from build123d import *

# Parameters (mm, degrees)
F1_DEPTH       = 260
F3_D           = 11
F3_DEPTH       = 30
F3_CBORE_D     = 19
F3_CBORE_DEPTH = 13
F3_TIP         = 3.3047334047
F4_D           = 8.8
F4_DEPTH       = 30
F4_TIP         = 2.6437867237
F5_D           = 11
F5_DEPTH       = 30
F5_TIP         = 3.3047334047


with BuildPart() as f1:
    # F0 (on Front) → F1 (new body)
    with BuildSketch(Plane.XZ):
        Polygon((100, 23), (0, 23), (0, 0), (95, 0), (95, -5), (100, -5), align=None)
    extrude(amount=-F1_DEPTH)

    # F3
    with Locations(Plane.XY.offset(23)):
        with Locations((14, 239), (86, 239), (14, 187), (86, 187), (86, 73), (86, 21), (14, 73), (14, 21)):
            CounterBoreHole(F3_D / 2, F3_CBORE_D / 2, F3_CBORE_DEPTH, depth=F3_DEPTH)
            with Locations((0, 0, -(F3_DEPTH + F3_TIP / 2))):  # 118° drill point
                Cone(0, F3_D / 2, F3_TIP, mode=Mode.SUBTRACT)

    # F4
    with Locations(Plane.XY.offset(23)):
        with Locations((31, 20), (69, 20), (31, 90), (69, 90), (31, 130), (69, 130)):
            Hole(F4_D / 2, depth=F4_DEPTH)
            with Locations((0, 0, -(F4_DEPTH + F4_TIP / 2))):  # 118° drill point
                Cone(0, F4_D / 2, F4_TIP, mode=Mode.SUBTRACT)

    # F5
    with Locations(Plane.XY.offset(23)):
        with Locations((9, 220), (91, 220), (91, 165), (9, 165)):
            Hole(F5_D / 2, depth=F5_DEPTH)
            with Locations((0, 0, -(F5_DEPTH + F5_TIP / 2))):  # 118° drill point
                Cone(0, F5_D / 2, F5_TIP, mode=Mode.SUBTRACT)


solid = f1.part
Source: CAD feature listing. Evaluate the final solid. Frame: model axes, mm. A direction names the side the tool comes from. Give positions to 0.01 mm unless a question says otherwise; leave off trailing zeros. Order: outer loops, then holes, each group sorted by start corner. A loop starts at its lowest first (then second) coordinate and runs counter-clockwise, first axis right, second up. Notation, with made-up numbers: (-7, 51.5) -> (40, 51.5) arc R24 cw to (40, 84.5) -> close; hole circle Ø7 at (38.5, -33.75). An arc over 180 degrees is marked (long way). Write item = value, one per line.
Item 1: Set-up query: faces 1 (the face through (95.061, 23.854, 16.591)), 2 (the face through (90.4, 183.7, 4.9)). Return all of +Z, -Z, +X, -X, +Y, -Y with unobstructed straight access to the full face (end or side cutting, diameter ignored); none if empty.
Check result:
face_1 = +Z
face_2 = +Z, -Z
Item 2: Mould query, pull axis X, two halves, no side actions, for faces 3 (the face through (100, 128, 9)), 4 (the face through (51, 128, 23)), 5 (the face through (96.495, 220.242, 11.915)). Classes: +X half, -X half, draft (parallel to the pull), parting line (faces both ways), or undercut.
Check result:
face_3 = +X half
face_4 = draft
face_5 = undercut
Item 3: Section query A-A (z = 16.75). State how many separate pieces and enclosed holes the cut face has, then the cut area to 3 significant figures.
Check result:
separate_pieces = 1
enclosed_holes = 18
area = 23,000 mm²
Item 4: Section query C-C (x = 31). Output: boundary loops of the cut face in (y, z), then the cut area to 3 significant figures.
Check result:
outline = (0, 0) -> (15.6, 0) -> (15.6, 23) -> (0, 23) -> close; (24.4, 0) -> (85.6, 0) -> (85.6, 23) -> (24.4, 23) -> close; (94.4, 0) -> (125.6, 0) -> (125.6, 23) -> (94.4, 23) -> close; (134.4, 0) -> (260, 0) -> (260, 23) -> (134.4, 23) -> close
area = 5,370 mm²
Item 5: Ray query, probe 1 along Y at (x, z) = (69, 7.75); probe 2 along X at (y, z) = (88, 9.75); probe 3 along X at (y, z) = (193.5, 21.25). Return the intervals inside material, ascending.
Check result:
probe_1 = 0 to 15.6, 24.4 to 85.6, 94.4 to 125.6, 134.4 to 260
probe_2 = 0 to 27.08, 34.92 to 65.08, 72.92 to 100
probe_3 = 0 to 7.07, 20.93 to 79.07, 92.93 to 100
Item 6: Section query B-B (y = 187). Output: boundary loops of the cut face in (x, z), then the cut area to 3 significant figures.
Check result:
outline = (0, 0) -> (8.5, 0) -> (8.5, 10) -> (4.5, 10) -> (4.5, 23) -> (0, 23) -> close; (19.5, 0) -> (80.5, 0) -> (80.5, 10) -> (76.5, 10) -> (76.5, 23) -> (23.5, 23) -> (23.5, 10) -> (19.5, 10) -> close; (91.5, 0) -> (95, 0) -> (95, -5) -> (100, -5) -> (100, 23) -> (95.5, 23) -> (95.5, 10) -> (91.5, 10) -> close
area = 1,610 mm²
Item 7: Contact query for flat-ended pins moving along their axis: pin 1 (21 mm diameter, centred on x = 10, y = 243, fed in from +Z); pin 2 (8 mm diameter, centred on x = 84, y = 142, fed in from -Z); pin 3 (5.5 mm diameter, centred on x = 89, y = 238.5, fed in from +Z). Output: stop coordinate, or through.
Check result:
pin_1 = 23
pin_2 = 0
pin_3 = 10
Item 8: Section query D-D (y = 156). Output: boundary loops of the cut face in (x, z), then the cut area to 4 significant figures.
Check result:
outline = (0, 0) -> (95, 0) -> (95, -5) -> (100, -5) -> (100, 23) -> (0, 23) -> close
area = 2,325 mm²
